Part print with two shaded views. Sizes in mm from the minimum x, y, z corner. Give positions to 0.01 mm unless a question says otherwise; leave off trailing zeros. Write each loop counter-clockwise with the first axis right and the second up, starting at its lowest first coordinate (ties: lowest second). Pieces come first, ordered by that corner, then holes. Notation, with made-up numbers: M 23,14.5 L 61,14.5 A20 cw 61,34.5 Z; hole C 77,49 d11. An arc over 180 degrees is marked long. One line per item, written item: value. Start each with the question number.
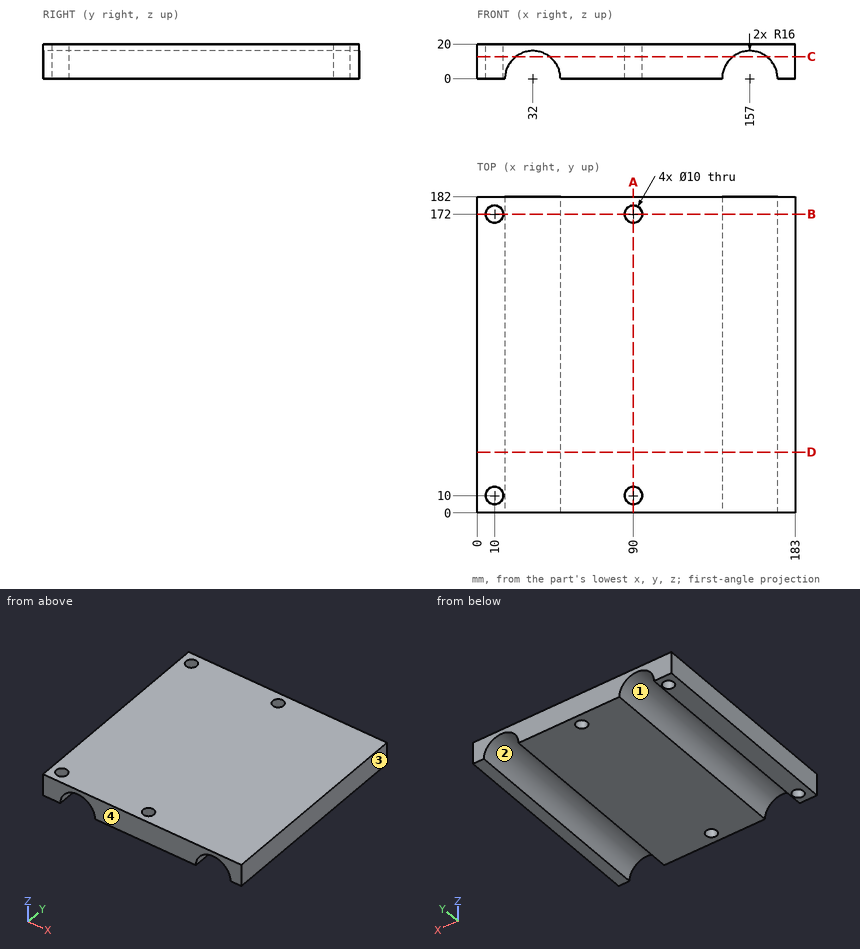
1) Band-saw the part on A-A (x = 90). List the corners of the cut face in (y, z).
2) Band-saw the part on B-B (y = 172). List the corners of the cut face in (x, z).
3) Probe line 1 along Y through (x, z) = (10, 5.75); line 2 along X through (y, z) = (36.5, 14); line 3 along X through (y, z) = (116, 5.75). List the from-to ranges inside material, lowest first. Write a range as from..to.
4) Band-saw the part on D-D (y = 35). List the corners of the cut face in (x, z), then the cut area to 3 significant figures.
5) Mould opens along X. For the marked faces 1, 2, 3 and 4 say: released by +X, released by -X, zero draft, split by the parting line, or undercut.
6) Band-saw the part on C-C (z = 12.75). List the corners of the cut face in (x, y), then the cut area to 3 significant figures.
Model answer:
1. outline: M 0,0 L 5,0 L 5,20 L 0,20 Z; M 15,0 L 167,0 L 167,20 L 15,20 Z; M 177,0 L 182,0 L 182,20 L 177,20 Z
2. outline: M 0,0 L 5,0 L 5,20 L 0,20 Z; M 15,0 L 16,0 A16 cw 48,0 L 85,0 L 85,20 L 15,20 Z; M 95,0 L 141,0 A16 cw 173,0 L 183,0 L 183,20 L 95,20 Z
3. line 1: y = 0..5, 15..167, 177..182
3. line 2: x = 0..24.25, 39.75..149.25, 164.75..183
3. line 3: x = 0..17.07, 46.93..142.07, 171.93..183
4. outline: M 0,0 L 16,0 A16 cw 48,0 L 141,0 A16 cw 173,0 L 183,0 L 183,20 L 0,20 Z
4. area: 2,860 mm²
5. face 1: undercut
5. face 2: undercut
5. face 3: released by +X
5. face 4: zero draft
6. outline: M 0,0 L 22.33,0 L 22.33,182 L 0,182 Z; M 41.67,0 L 147.33,0 L 147.33,182 L 41.67,182 Z; M 166.67,0 L 183,0 L 183,182 L 166.67,182 Z; hole C 10,10 d10; hole C 10,172 d10; hole C 90,10 d10; hole C 90,172 d10
6. area: 26,000 mm²
